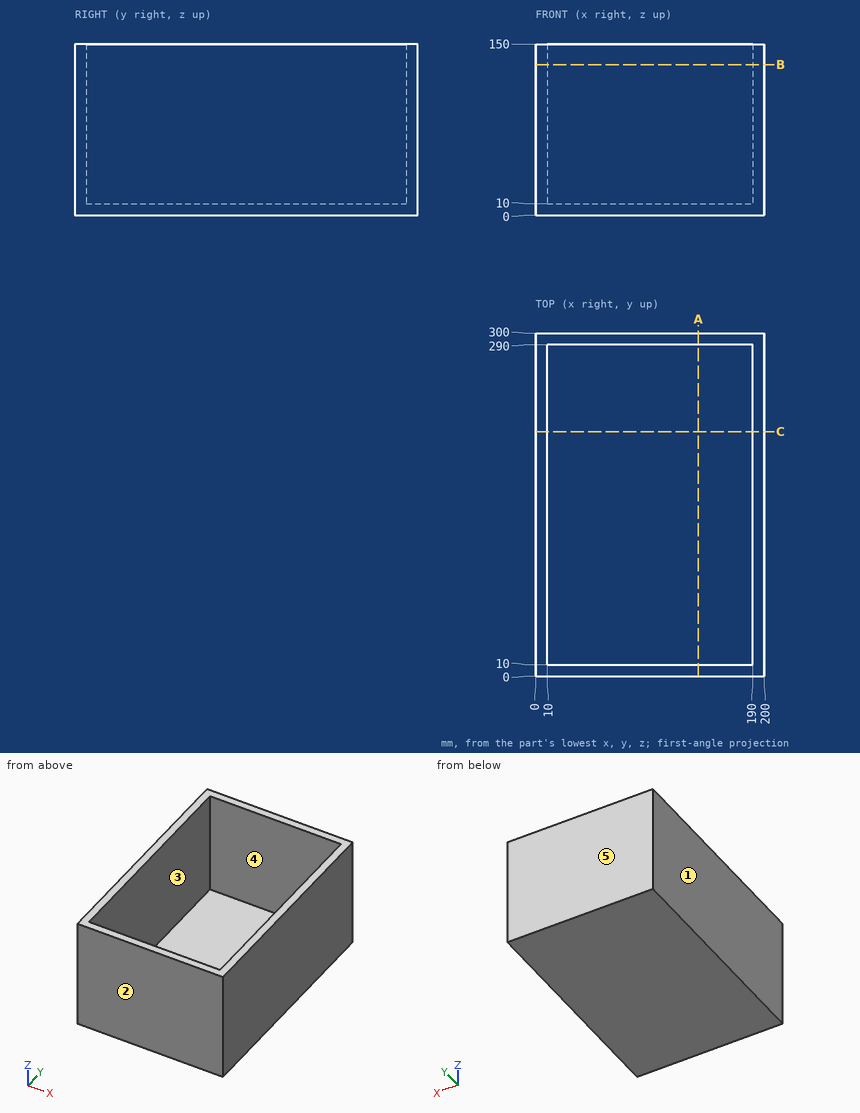
Geometry check sheet. Reference: drawing and pictorial views, mm from the part's lowest x, y, z. A direction names the side the tool comes from. Round coordinates to 2 decimals unless told otherwise and drop trailing zeros. Loops run counter-clockwise (first coordinate to the right, second up) from the corner with the lowest first, then second, coordinate; pieces in that order, holes last. Notation, with made-up numbers: (-28, -12) -> (-2, -12) arc R22 ccw to (-2, 20) -> close; hole circle Ø11 at (-8, 19.25). An arc over 180 degrees is marked (long way). Answer as a JSON object with one key per item and string values. Group by question number.
Item 1: Cross-section at B-B, the plane z = 132. Record the cut outline in (x, y), plus the area to 3 significant figures.
Item 2: Thickness scan on line 1 along X through (y, z) = (185, 78); line 2 along Y through (x, z) = (45.5, 123); line 3 along Z through (x, y) = (13, 235). Record the ranges inside material, lowest first.
Item 3: Set-up check for the marked faces 4 and 5: record each of +Z, -Z, +X, -X, +Y, -Y from which the full face is reachable in a straight line by a thin tool's end or side.
Item 4: Release check for a two-part mould opening along Y. For the marked faces 1, 2 and 3 record: pulls with the +Y half, pulls with the -Y half, needs draft (parallel to the pull), parting line crosses it, or undercut.
Item 5: Cross-section at A-A, the plane x = 142.5. Record the cut outline in (y, z), plus the area to 3 significant figures.
Item 6: Depth check by flat-ended pin: pin 1 Ø4 at (x, y) = (24.5, 70) entering from +Z; pin 2 Ø1.5 at (x, z) = (94.5, 122) entering from -Y. Enter the tip coordinate at first touch or a pass-through.
Item 7: Cross-section at C-C, the plane y = 214. Record the cut outline in (x, z), plus the area to 3 significant figures.
Determined:
{
 "1": {"outline": "(0, 0) -> (200, 0) -> (200, 300) -> (0, 300) -> close; hole (10, 10) -> (190, 10) -> (190, 290) -> (10, 290) -> close", "area": "9,600 mm²"},
 "2": {"line 1": "x = 0 to 10, 190 to 200", "line 2": "y = 0 to 10, 290 to 300", "line 3": "z = 0 to 10"},
 "3": {"face 4": "+Z", "face 5": "+Z, -Z, +X, -X, +Y"},
 "4": {"face 1": "needs draft", "face 2": "pulls with the -Y half", "face 3": "undercut"},
 "5": {"outline": "(0, 0) -> (300, 0) -> (300, 150) -> (290, 150) -> (290, 10) -> (10, 10) -> (10, 150) -> (0, 150) -> close", "area": "5,800 mm²"},
 "6": {"pin 1": "stops at z = 10", "pin 2": "stops at y = 0"},
 "7": {"outline": "(0, 0) -> (200, 0) -> (200, 150) -> (190, 150) -> (190, 10) -> (10, 10) -> (10, 150) -> (0, 150) -> close", "area": "4,800 mm²"}
}
